from build123d import *

# Parameters (mm, degrees)
F0_W     = 30
F0_H     = 30
F0_R     = 10.75
F1_DEPTH = 3
F2_DEPTH = 0.6
F3_R     = 0.3


with BuildPart() as f1:
    # F0 (on Top) → F1 (new body)
    with BuildSketch(Plane.XY):
        Rectangle(F0_W, F0_H)
        Circle(F0_R, mode=Mode.SUBTRACT)
    extrude(amount=F1_DEPTH)

    # F0 (on Top) → F2 (join)
    with BuildSketch(Plane.XY):
        Circle(F0_R)
    extrude(amount=F2_DEPTH)

    # F3
    f3_edges = [f1.edges().sort_by_distance(p)[0] for p in [
        (-10.75, 0, 3),
    ]]
    fillet(f3_edges, radius=F3_R)


solid = f1.part
Work out the finished part from the listing and answer in its coordinate system (mm). A direction names the side the tool comes from. Coordinates: 2 decimals unless noted, no trailing zeros. Write each loop counter-clockwise with the first axis right and the second up, starting at its lowest first coordinate (ties: lowest second). Pieces come first, ordered by that corner, then holes.
1. Consider line 1 along Y through (x, z) = (0, 2.3); line 2 along X through (y, z) = (7, 1.4); line 3 along Y through (x, z) = (6.25, 0.9). Determine where each line is inside the solid, lowest interval first.
Results list:
line 1: y = -15 to -10.75, 10.75 to 15
line 2: x = -15 to -8.16, 8.16 to 15
line 3: y = -15 to -8.75, 8.75 to 15
2. The part is cut by section A-A, the plane z = 2.1. Write down the section's boundary in (x, y), and give its area (3 significant figures).
Results list:
outline: (-15, -15) - (15, -15) - (15, 15) - (-15, 15) - close; hole circle Ø21.5 at (0, 0)
area: 537 mm2
3. For a pull along X with two mould halves and no side action, classify faces 1 (the flat face through (15, 0, 1)), 2 (the flat face through (0, 0, 0.6)), 3 (the flat face through (-15, 0, 1)) as +X half, -X half, draft (parallel to the pull), parting line (faces both ways), or undercut.
Results list:
face 1: +X half
face 2: undercut
face 3: -X half
4. For faces 4 (the cylindrical face through (-1.4, 10.66, 1.64)), 5 (the flat face through (0, 15, 1)), determine the directions among +Z, -Z, +X, -X, +Y, -Y from which every point of the face is accessible in a straight line to the end or side of a thin tool.
Results list:
face 4: +Z
face 5: +Z, -Z, +X, -X, +Y
5. The part is cut by section B-B, the plane y = 0. Write down the section's boundary in (x, z).
Results list:
outline: (-15, 0) - (15, 0) - (15, 3) - (11.05, 3) arc R0.3 ccw to (10.75, 2.7) - (10.75, 0.6) - (-10.75, 0.6) - (-10.75, 2.7) arc R0.3 ccw to (-11.05, 3) - (-15, 3) - close
